Source: CAD feature listing. Evaluate the final solid. Frame: model axes, mm. Face numbers are marked on the shaded views. Coordinates: 2 decimals unless noted, no trailing zeros. Order: outer loops, then holes, each group sorted by start corner. A loop starts at its lowest first (then second) coordinate and runs counter-clockwise, first axis right, second up. Notation, with made-up numbers: (-22, 10) -> (16, 10) arc R5 ccw to (16, 18) -> close; hole circle Ø3 at (73, 83.25). An arc over 180 degrees is marked (long way). Write each question's results on one line, items separated by ' | '. Start each with the question number.
from build123d import *

# Parameters (mm, degrees)
SKETCH3_R           = 12.7381
SKETCH3_R_2         = 9.5631
BOSS_EXTRUDE1_DEPTH = 12.7
SKETCH4_R           = 14.2875
SKETCH4_R_2         = 12.7381
BOSS_EXTRUDE2_DEPTH = 3.175
CHAMFER1_SIZE       = 0.191262
FILLET1_R           = 0.1783334


with BuildPart() as part:
    # Sketch3 → Boss-Extrude1 (new body)
    with BuildSketch(Plane.XY):
        Circle(SKETCH3_R)
        Circle(SKETCH3_R_2, mode=Mode.SUBTRACT)
    extrude(amount=BOSS_EXTRUDE1_DEPTH)

    # Sketch4 → Boss-Extrude2 (add)
    with BuildSketch(Plane.XY):
        Circle(SKETCH4_R)
        Circle(SKETCH4_R_2, mode=Mode.SUBTRACT)
    extrude(amount=BOSS_EXTRUDE2_DEPTH)

    # Chamfer1
    chamfer1_edges = [part.edges().sort_by_distance(p)[0] for p in [
        (-9.5631, 0, 0),
        (-9.5631, 0, 12.7),
    ]]
    chamfer(chamfer1_edges, length=CHAMFER1_SIZE)

    # Fillet1
    fillet1_edges = [part.edges().sort_by_distance(p)[0] for p in [
        (-14.2875, 0, 3.175),
        (-14.2875, 0, 0),
        (-12.7381, 0, 3.175),
        (-12.7381, 0, 12.7),
    ]]
    fillet(fillet1_edges, radius=FILLET1_R)


solid = part.part
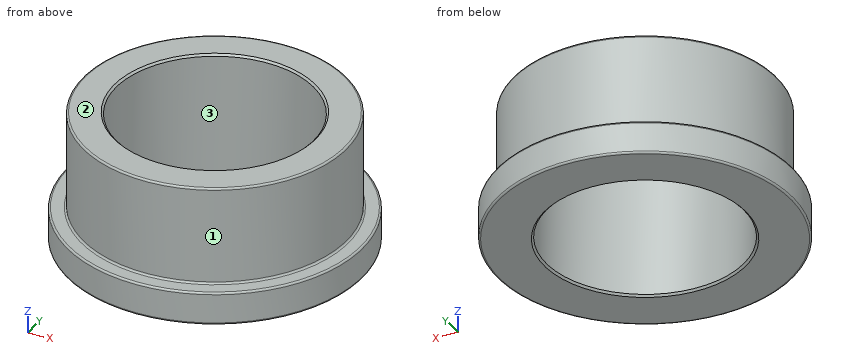
(1) Line query: L1, parallel to Y at x = 0, z = 9.5; L2, parallel to Y at x = 6.5, z = 9.5. Output: solid intervals per line, ascending.
(2) First-contact query: P1, Ø1.5, axis at y = 2, z = 3.5, coming from the -X side; P2, Ø1, axis at y = -6, z = 3.5, coming from the +X side; P3, Ø6, axis at x = 8.5, z = 6.5, coming from the -Y side. Flat tips, straight axial feed; report the tip coordinate or a pass-through.
(3) Section C-C on z = 2.5. Return the cut outline in (x, y) (1 decimal), then the cut area to 3 significant figures.
(4) Draft query along Y for the marked faces 1, 2 and 3. Return one class per face: released by +Y, released by -Y, zero draft, split by the parting line, or undercut.
Results list:
1) L1: y = -12.74 to -9.56, 9.56 to 12.74 | L2: y = -10.95 to -7.01, 7.01 to 10.95
2) P1: stops at x = -14.22 | P2: stops at x = 13.07 | P3: stops at y = -11.49
3) outline: circle Ø28.6 at (0, 0); hole circle Ø19.1 at (0, 0) | area: 354 mm²
4) face 1: split by the parting line | face 2: zero draft | face 3: undercut
